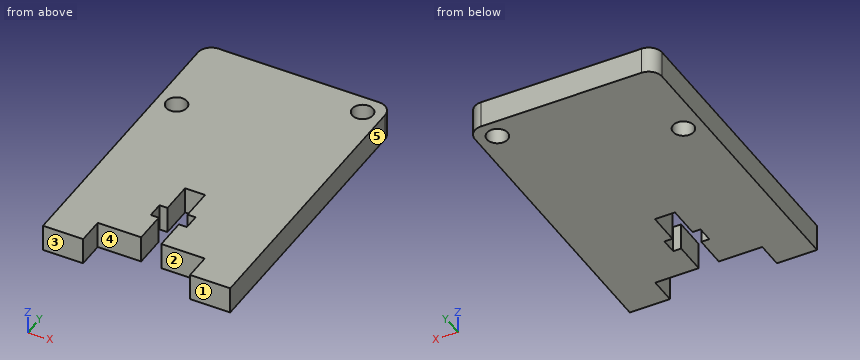
Autodesk Inventor part; units mm, degrees
ref_plane "YZ Plane" through (0, 0, 0) normal (1, 0, 0) x (0, 1, 0)
ref_plane "XZ Plane" through (0, 0, 0) normal (0, 1, 0) x (-1, 0, 0)
ref_plane "XY Plane" through (0, 0, 0) normal (0, 0, 1) x (1, 0, 0)
sketch "Sketch1" plane through (0, 0, 0) normal (0, 0, 1) x (1, 0, 0)
  line L0 (-14, 0) -> (14, 0)
  line L1 (14, 0) -> (14, 16)
  line L2 (14, 16) -> (-14, 16)
  line L3 (-14, 16) -> (-14, 0)
  circle A0 centre (-11.1, 2.85) radius 1.55
  circle A1 centre (11.1, 13.15) radius 1.55
  line L4 (-11.1, 2.85) -> (-14, 2.85) construction
  line L5 (11.1, 13.15) -> (14, 13.15) construction
  line L6 (11.1, 13.15) -> (11.1, 16) construction
  line L7 (-11.1, 2.85) -> (-11.1, 0) construction
  line L8 (-14, 0) -> (14, 0) construction
  line L9 (14, 0) -> (14, -24.4)
  line L10 (14, -24.4) -> (8, -24.4) construction
  line L11 (-14, -24.4) -> (-14, 0)
  line L12 (-14, -24.4) -> (-8, -24.4) construction
  line L13 (-8, -24.4) -> (-8, -28.4)
  line L14 (-8, -28.4) -> (-14, -28.4)
  line L15 (-14, -28.4) -> (-14, -24.4)
  line L16 (14, -24.4) -> (8, -24.4) construction
  line L17 (8, -24.4) -> (8, -28.4)
  line L18 (8, -28.4) -> (14, -28.4)
  line L19 (14, -28.4) -> (14, -24.4)
  line L20 (-8, -24.4) -> (-14, -24.4) construction
  line L21 (8, -24.4) -> (-8, -24.4)
  point P0 (0, 0)
  point P1 (0, 0)
  point P2 (14, 0)
  point P3 (14, 0)
  dimension "d0" = 3.1
  dimension "d1" = 22.2
  dimension "d2" = 10.3
  dimension "d3" = 16
  dimension "d4" = 28
  dimension "d5" = 40.4
  dimension "d8" = 6
  dimension "d9" = 6
  dimension "d10" = 4
extrude "Extrusion1" add sketch "Sketch1" along normal blind 4
sketch "Sketch2" plane through (0, 0, 4) normal (0, 0, 1) x (1, 0, 0)
  line L0 (14, -28.4) -> (14, 16) construction
  line L1 (14, 16) -> (-14, 16) construction
  line L2 (-14, 16) -> (-14, -28.4) construction
  line L3 (-14, -28.4) -> (-8, -28.4) construction
  line L4 (-8, -28.4) -> (-8, -24.4) construction
  line L5 (-8, -24.4) -> (8, -24.4) construction
  line L6 (8, -24.4) -> (8, -28.4) construction
  line L7 (8, -28.4) -> (14, -28.4) construction
  circle A0 centre (-11.1, 2.85) radius 1.55 construction
  circle A1 centre (11.1, 13.15) radius 1.55 construction
  line L8 (-1.5, -24.4) -> (1.5, -24.4)
  line L9 (1.5, -24.4) -> (1.5, -12.4)
  line L10 (1.5, -12.4) -> (-1.5, -12.4)
  line L11 (-1.5, -12.4) -> (-1.5, -24.4)
  line L12 (-2.7, -19.6) -> (2.7, -19.6)
  line L13 (2.7, -19.6) -> (2.7, -17.2)
  line L14 (2.7, -17.2) -> (-2.7, -17.2)
  line L15 (-2.7, -17.2) -> (-2.7, -19.6)
  point P0 (0, 0)
  point P1 (-2.7, -18.4)
  point P2 (-1.5, -18.4)
  point P3 (0, -17.2)
  point P4 (0, -12.4)
  point P5 (0, -24.4)
  point P6 (0, -24.4)
  point P7 (-1.5, -19.6)
  point P8 (1.5, -19.6)
  point P9 (1.5, -17.2)
  point P10 (-1.5, -17.2)
  dimension "d11" = 3
  dimension "d12" = 2.4
  dimension "d13" = 5.4
  dimension "d14" = 12
extrude "Extrusion2" cut sketch "Sketch2" against normal up to next
fillet "Fillet1" radius 2 2 edges at (14, 16, 2) (-14, 16, 2)
properties part number "SwitchHolder_Bottom_V3" material "MDF Medium Density Fiberboard"
CAD build for the part. Positions are in the model's coordinates, mm. Face numbers are marked on the shaded views. A direction names the side the tool comes from. Give positions to 0.01 mm unless a question says otherwise; leave off trailing zeros. Write each loop counter-clockwise with the first axis right and the second up, starting at its lowest first coordinate (ties: lowest second). Pieces come first, ordered by that corner, then holes. Notation, with made-up numbers: M -26.75,59 L -12.75,59 A30 ccw -12.75,85 Z; hole C -28,37 d1. An arc over 180 degrees is marked long. Put each result on its own line as item: value. Start each with the question number.
(1) Band-saw the part on A-A, the plane x = -11.1. Write the cut outline in (y, z).
(2) Flat gauge pins, fed straight in: pin 1 Ø1.9 at (x, y) = (-11.1, 2.85) entering from -Z; pin 2 Ø2 at (x, y) = (1, -23) entering from +Z; pin 3 Ø1.3 at (x, z) = (2, 3) entering from -Y. Where does each tip first touch, or does it go through?
(3) Band-saw the part on D-D, the plane x = -5.5. Write the cut outline in (y, z), and give its area (3 significant figures).
(4) Mould opens along X. For the marked faces 3, 4 and 5 say: +X half, -X half, draft (parallel to the pull), parting line (faces both ways), or undercut.
(5) Band-saw the part on B-B, the plane z = 3.3. Write the cut outline in (x, y), and give its area (3 significant figures).
(6) Probe L1, parallel to X at y = -23.5, z = 0.8; L2, parallel to Y at x = -11.1, z = 1.7; L3, parallel to Y at x = 11.1, z = 2.65. List the from-to ranges inside material, lowest first.
(7) Which spindle directions (+Z, -Z, +X, -X, +Y, -Y) get a long thin tool onto all of the face, cutting with end or side? Do the marked faces 1 and 2. Say none if no direction does.
(8) Band-saw the part on C-C, the plane y = 2.85. Write the cut outline in (x, z).
Response values:
1. outline: M -28.4,0 L 1.3,0 L 1.3,4 L -28.4,4 Z; M 4.4,0 L 16,0 L 16,4 L 4.4,4 Z
2. pin 1: passes through
2. pin 2: stops at z = 4
2. pin 3: stops at y = -24.4
3. outline: M -24.4,0 L 16,0 L 16,4 L -24.4,4 Z
3. area: 162 mm2
4. face 3: draft
4. face 4: undercut
4. face 5: +X half
5. outline: M -14,-28.4 L -8,-28.4 L -8,-24.4 L -1.5,-24.4 L -1.5,-19.6 L -2.7,-19.6 L -2.7,-17.2 L -1.5,-17.2 L -1.5,-12.4 L 1.5,-12.4 L 1.5,-17.2 L 2.7,-17.2 L 2.7,-19.6 L 1.5,-19.6 L 1.5,-24.4 L 8,-24.4 L 8,-28.4 L 14,-28.4 L 14,14 A2 ccw 12,16 L -12,16 A2 ccw -14,14 Z; hole C -11.1,2.85 d3.1; hole C 11.1,13.15 d3.1
5. area: 1,120 mm2
6. L1: x = -14 to -1.5, 1.5 to 14
6. L2: y = -28.4 to 1.3, 4.4 to 16
6. L3: y = -28.4 to 11.6, 14.7 to 16
7. face 1: +Z, -Z, +X, -X, -Y
7. face 2: +Z, -Z, -Y
8. outline: M -14,0 L -12.65,0 L -12.65,4 L -14,4 Z; M -9.55,0 L 14,0 L 14,4 L -9.55,4 Z
